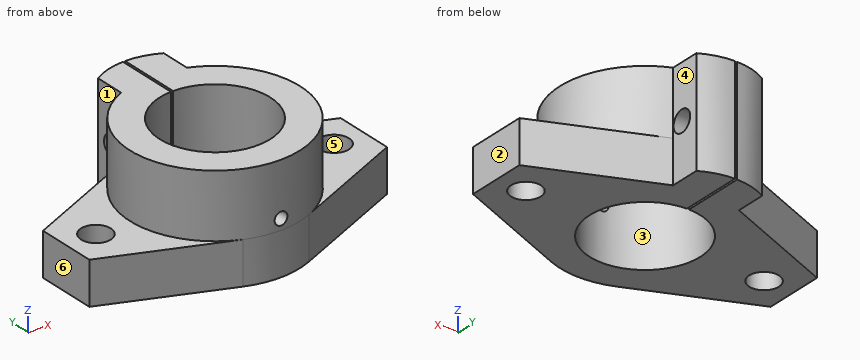
from build123d import *

# Parameters (mm, degrees)
SKETCH_1_R          = 3.5
SKETCH_1_R_2        = 13
EXTRUDE_2_DEPTH     = 10
SKETCH_2_R          = 13
EXTRUDE_3_DEPTH     = 15
SKETCH_3_W          = 0.517195108
SKETCH_3_H          = 18.726193104
CUT_EXTRUDE_1_DEPTH = 26
SKETCH_4_R          = 2.5
CUT_EXTRUDE_2_DEPTH = 43.740275714
SKETCH_5_R          = 1.5
CUT_EXTRUDE_3_DEPTH = 21


with BuildPart() as part:
    # 草图1 → 凸台-拉伸2 (new body)
    with BuildSketch(Plane.XY):
        with BuildLine():
            Line((-35, -7), (-7.740275714, -18.44147857))
            ThreePointArc((-7.740275714, -18.44147857), (0, -20), (7.740275714, -18.44147857))
            Line((7.740275714, -18.44147857), (35, -7))
            Line((35, -7), (35, 7))
            Line((35, 7), (7.740275714, 18.44147857))
            Line((7.740275714, 18.44147857), (7.740275714, 25.44147857))
            ThreePointArc((7.740275714, 25.44147857), (0, 27.494244152), (-7.740275714, 25.44147857))
            Line((-7.740275714, 25.44147857), (-7.740275714, 18.44147857))
            Line((-7.740275714, 18.44147857), (-35, 7))
            Line((-35, 7), (-35, -7))
        make_face()
        with Locations((-28, 0)):
            Circle(SKETCH_1_R, mode=Mode.SUBTRACT)
        Circle(SKETCH_1_R_2, mode=Mode.SUBTRACT)
        with Locations((28, 0)):
            Circle(SKETCH_1_R, mode=Mode.SUBTRACT)
    extrude(amount=EXTRUDE_2_DEPTH)

    # 草图2 → 凸台-拉伸3 (add)
    with BuildSketch(Plane.XY.offset(10)):
        with BuildLine():
            Line((-7.740275714, 18.44147857), (-7.740275714, 25.44147857))
            ThreePointArc((-7.740275714, 25.44147857), (0, 27.494244152), (7.740275714, 25.44147857))
            Line((7.740275714, 25.44147857), (7.740275714, 18.44147857))
            ThreePointArc((7.740275714, 18.44147857), (0, -20), (-7.740275714, 18.44147857))
        make_face()
        Circle(SKETCH_2_R, mode=Mode.SUBTRACT)
    extrude(amount=EXTRUDE_3_DEPTH)

    # 草图3 → 切除-拉伸1 (cut, through all)
    with BuildSketch(Plane.XY.offset(25)):
        with Locations((0, 21.741202931)):
            Rectangle(SKETCH_3_W, SKETCH_3_H)
    extrude(amount=-CUT_EXTRUDE_1_DEPTH, mode=Mode.SUBTRACT)

    # 草图4 → 切除-拉伸2 (cut, through all)
    with BuildSketch(Plane(origin=(7.740275714, 0, 0), x_dir=(0, 0, -1), z_dir=(1, 0, 0))):
        with Locations((-12.5, 21.086423576)):
            Circle(SKETCH_4_R)
    extrude(amount=-CUT_EXTRUDE_2_DEPTH, mode=Mode.SUBTRACT)

    # 草图5 → 切除-拉伸3 (cut, through all)
    with BuildSketch(Plane(origin=(0, 0, 0), x_dir=(1, 0, 0), z_dir=(0, 1, 0))):
        with Locations((0, -12.5)):
            Circle(SKETCH_5_R)
    extrude(amount=-CUT_EXTRUDE_3_DEPTH, mode=Mode.SUBTRACT)


solid = part.part
CAD build for the part. Positions are in the model's coordinates, mm. Face numbers are marked on the shaded views. A direction names the side the tool comes from. Give positions to 0.01 mm unless a question says otherwise; leave off trailing zeros. Write each loop counter-clockwise with the first axis right and the second up, starting at its lowest first coordinate (ties: lowest second). Pieces come first, ordered by that corner, then holes. Notation, with made-up numbers: (58.5, -26) - (100.5, -26) arc R19 cw to (100.5, 7) - close; hole circle Ø10 at (-8, 10). An arc over 180 degrees is marked (long way). Put each result on its own line as item: value.
(1) Drop flat-ended pins along their axis: pin 1 Ø6 at (x, z) = (-10, 21.5) entering from -Y (3 decimals); pin 2 Ø6 at (y, z) = (21.09, 12.5) entering from -X; pin 3 Ø5.5 at (y, z) = (20.5, 8) entering from +X; pin 4 Ø4.5 at (y, z) = (21.09, 12.5) entering from -X. Give the stop position or say it passes through.
Working result:
pin 1: y = -18.735
pin 2: x = -8.53
pin 3: x = 9.39
pin 4: through
(2) Saw through at A-A (y = 0). List the corners of the cut face in (x, z), then the cut area to 3 significant figures.
Working result:
outline: (-35, 0) - (-31.5, 0) - (-31.5, 10) - (-35, 10) - close; (-24.5, 0) - (-13, 0) - (-13, 25) - (-20, 25) - (-20, 10) - (-24.5, 10) - close; (13, 0) - (24.5, 0) - (24.5, 10) - (20, 10) - (20, 25) - (13, 25) - close; (31.5, 0) - (35, 0) - (35, 10) - (31.5, 10) - close
area: 510 mm^2
(3) Pull direction X, two halves, no side cores. Call the marked faces 3, 4, 5 and 6: released by +X, released by -X, zero draft, split by the parting line, or undercut.
Working result:
face 3: undercut
face 4: released by +X
face 5: undercut
face 6: released by -X
(4) Saw through at C-C (x = -28). List the corners of the cut face in (y, z).
Working result:
outline: (-9.94, 0) - (-3.5, 0) - (-3.5, 10) - (-9.94, 10) - close; (3.5, 0) - (9.94, 0) - (9.94, 10) - (3.5, 10) - close
(5) Saw through at D-D (z = 17.5). List the corners of the cut face in (x, y), then the cut area to 3 significant figures.
Working result:
outline: (-7.74, 18.44) arc R20 ccw (long way) to (7.74, 18.44) - (7.74, 25.44) arc R15.62 ccw to (0.26, 27.49) - (0.26, 13) arc R13 cw (long way) to (-0.26, 13) - (-0.26, 27.49) arc R15.62 ccw to (-7.74, 25.44) - close
area: 832 mm^2
(6) Tool access for the marked faces 1 and 2: list every direction of +Z, -Z, +X, -X, +Y, -Y with a clear straight run to the whole face (end or side of a thin tool).
Working result:
face 1: +Z, -Z, -X, +Y
face 2: +Z, -Z, +X, +Y, -Y
(7) Wall check: L1, parallel to Y at x = -5.5, z = 12.5; L2, parallel to X at y = 18.5, z = 19.5; L3, parallel to Y at x = -3.25, z = 12.5. Give the ranges that are in metal, low to high.
Working result:
L1: -19.23 to -11.78, 11.78 to 18.59, 23.59 to 26.49
L2: -7.74 to -0.26, 0.26 to 7.74
L3: -19.73 to -12.59, 12.59 to 18.59, 23.59 to 27.15
(8) Saw through at B-B (z = 12.5). List the corners of the cut face in (x, y).
Working result:
outline: (-7.74, 18.44) arc R20 ccw to (-1.5, -19.94) - (-1.5, -12.91) arc R13 cw to (-0.26, 13) - (-0.26, 18.59) - (-7.74, 18.59) - close; (-7.74, 23.59) - (-0.26, 23.59) - (-0.26, 27.49) arc R15.62 ccw to (-7.74, 25.44) - close; (0.26, 13) arc R13 cw to (1.5, -12.91) - (1.5, -19.94) arc R20 ccw to (7.74, 18.44) - (7.74, 18.59) - (0.26, 18.59) - close; (0.26, 23.59) - (7.74, 23.59) - (7.74, 25.44) arc R15.62 ccw to (0.26, 27.49) - close
